Geometry: final body of the model. Coordinates: model frame, mm. A direction names the side the tool comes from. Round coordinates to 2 decimals unless told otherwise and drop trailing zeros. Order: outer loops, then holes, each group sorted by start corner. A loop starts at its lowest first (then second) coordinate and runs counter-clockwise, first axis right, second up. Notation, with made-up numbers: (71.5, -10.5) - (101.5, -10.5) arc R25 cw to (101.5, 20.5) - close; hole circle Ø11 at (12, -24). An arc over 180 degrees is marked (long way). Put each result on its own line as item: value. Start each with the question number.
(1) Section A-A (x = 0). Count the separate pieces of the cut face and the enclosed holes in it, and give its area (3 significant figures).
(2) Material intervals for L1, parallel to X at y = 2.5, z = 0; L2, parallel to Y at x = -3.5, z = 7; L3, parallel to Y at x = 0, z = 14, sorted ascending. Write a range as [from, to].
(3) Section D-D (x = 8.75). Output: boundary loops of the cut face in (y, z), and give its area (3 significant figures).
(4) Pin query (flat end, axial travel): P1, Ø8, axis at x = 2.5, z = 24.5, coming from the -Y side; P2, Ø1.5, axis at y = 3, z = 16, coming from the -X side; P3, Ø10, axis at x = -3, z = 23, coming from the +Y side. Return the tip coordinate at first contact, or that it passes through.
(5) Pull-direction query (X, two-part tool) for faces 5 (the face through (0, 1, 20)), 6 (the face through (-0.05, 5.01, -5.19)), 7 (the face through (-5.19, 5.01, 0.05)); classes: released by +X, released by -X, zero draft, split by the parting line, or undercut.
(6) Section C-C (z = -7.5). Output: boundary loops of the cut face in (x, y), and give its area (3 significant figures).
(7) Section B-B (y = 4.75). Output: boundary loops of the cut face in (x, z), and give its area (3 significant figures).
(8) Access query for faces 1 (the face through (5.272, 4.986, 5.335)), 2 (the face through (-0.1, 0.5, 9.798)), 3 (the face through (5, 2, 18)), 4 (the face through (-5.335, 4.986, 5.272)). Directions: +Z, -Z, +X, -X, +Y, -Y. A direction counts if a zero-diameter tool reaches every point of the face in a straight line with its end or side. Return the directions, or none.
from build123d import *

# Parameters (mm, degrees)
SKETCH1_R           = 11
SKETCH1_R_2         = 4.25
BOSS_EXTRUDE1_DEPTH = 4
SKETCH2_R           = 1.4
CUT_EXTRUDE1_DEPTH  = 17.062378404
SKETCH3_R           = 7.5
BOSS_EXTRUDE2_DEPTH = 2
SKETCH4_R           = 2.811136831
CUT_EXTRUDE2_DEPTH  = 2
SKETCH5_R           = 4.5
BOSS_EXTRUDE3_DEPTH = 7
CUT_EXTRUDE3_START  = -6
SKETCH6_R           = 4.5
SKETCH6_R_2         = 4
CUT_EXTRUDE3_DEPTH  = 6
BOSS_EXTRUDE4_DEPTH = 4
SKETCH11_W          = 20
SKETCH11_H          = 1
CUT_EXTRUDE5_DEPTH  = 37.234215306
FILLET1_R           = 3


with BuildPart() as part:
    # Sketch1 → Boss-Extrude1 (new body)
    with BuildSketch(Plane(origin=(0, 0, 0), x_dir=(1, 0, 0), z_dir=(0, 1, 0))):
        with Locations(Location((0, 0, 0), (0, 0, 270))):
            Circle(SKETCH1_R)
        with Locations(Location((0, 0, 0), (0, 0, 270))):
            Circle(SKETCH1_R_2, mode=Mode.SUBTRACT)
    extrude(amount=BOSS_EXTRUDE1_DEPTH)

    # Sketch2 → Cut-Extrude1 (cut, through all)
    with BuildSketch(Plane(origin=(0, 4, 0), x_dir=(1, 0, 0), z_dir=(0, 1, 0))):
        with Locations(Location((0, 8, 0), (0, 0, 270))):
            Circle(SKETCH2_R)
        with Locations(Location((8, 0, 0), (0, 0, 270))):
            Circle(SKETCH2_R)
        with Locations(Location((0, -8, 0), (0, 0, 270))):
            Circle(SKETCH2_R)
        with Locations(Location((-8, 0, 0), (0, 0, 270))):
            Circle(SKETCH2_R)
    extrude(amount=-CUT_EXTRUDE1_DEPTH, mode=Mode.SUBTRACT)

    # Sketch3 → Boss-Extrude2 (add)
    with BuildSketch(Plane(origin=(0, 4, 0), x_dir=(1, 0, 0), z_dir=(0, 1, 0))):
        with Locations(Location((0, 0, 0), (0, 0, 80.315835906))):
            Circle(SKETCH3_R)
    extrude(amount=BOSS_EXTRUDE2_DEPTH)

    # Sketch4 → Cut-Extrude2 (cut)
    with BuildSketch(Plane(origin=(0, 6, 0), x_dir=(1, 0, 0), z_dir=(0, 1, 0))):
        with Locations((8, 0)):
            Circle(SKETCH4_R)
        with Locations((0, -8)):
            Circle(SKETCH4_R)
        with Locations((-8, 0)):
            Circle(SKETCH4_R)
        with Locations((0, 8)):
            Circle(SKETCH4_R)
    extrude(amount=-CUT_EXTRUDE2_DEPTH, mode=Mode.SUBTRACT)

    # Sketch5 → Boss-Extrude3 (add)
    with BuildSketch(Plane(origin=(0, 6, 0), x_dir=(1, 0, 0), z_dir=(0, 1, 0))):
        with Locations(Location((0, 0, 0), (0, 0, 270))):
            Circle(SKETCH5_R)
    extrude(amount=BOSS_EXTRUDE3_DEPTH)

    # Sketch6 → Cut-Extrude3 (cut)
    with BuildSketch(Plane(origin=(0, 13, 0), x_dir=(1, 0, 0), z_dir=(0, 1, 0)).offset(CUT_EXTRUDE3_START)):
        with Locations(Location((0, 0, 0), (0, 0, 270))):
            Circle(SKETCH6_R)
        with Locations(Location((0, 0, 0), (0, 0, 270))):
            Circle(SKETCH6_R_2, mode=Mode.SUBTRACT)
    extrude(amount=CUT_EXTRUDE3_DEPTH, mode=Mode.SUBTRACT)

    # Sketch8 → Boss-Extrude4 (add)
    with BuildSketch(Plane.XZ):
        with BuildLine():
            Line((5, 29.797958971), (-5, 29.797958971))
            Line((-5, 29.797958971), (-5, 9.797958971))
            ThreePointArc((-5, 9.797958971), (0, 11), (5, 9.797958971))
            Line((5, 9.797958971), (5, 29.797958971))
        make_face()
    extrude(amount=-BOSS_EXTRUDE4_DEPTH)

    # Sketch11 → Cut-Extrude5 (cut, through all)
    with BuildSketch(Plane.ZY.offset(5)):
        with Locations((19.797958971, 0.5)):
            Rectangle(SKETCH11_W, SKETCH11_H)
    extrude(amount=-CUT_EXTRUDE5_DEPTH, mode=Mode.SUBTRACT)

    # Fillet1
    fillet1_edges = [part.edges().sort_by_distance(p)[0] for p in [
        (5, 2.5, 29.797958971),
        (-5, 2.5, 29.797958971),
    ]]
    fillet(fillet1_edges, radius=FILLET1_R)


solid = part.part
Checks:
1. separate pieces: 3
1. enclosed holes: 0
1. area: 165 mm²
2. L1: x = [-11, -9.4], [-6.6, -4.25], [4.25, 6.6], [9.4, 11]
2. L2: y = [0, 4]
2. L3: y = [1, 4]
3. outline: (0, -6.67) - (4, -6.67) - (4, -1.18) - (0, -1.18) - close; (0, 1.18) - (4, 1.18) - (4, 6.67) - (0, 6.67) - close
3. area: 43.9 mm²
4. P1: stops at y = 1
4. P2: stops at x = -5
4. P3: stops at y = 4
5. face 5: zero draft
5. face 6: undercut
5. face 7: released by -X
6. outline: (-8.05, 0) - (-1.31, 0) - (-1.31, 4) - (-8.05, 4) - close; (1.31, 0) - (8.05, 0) - (8.05, 4) - (1.31, 4) - close
6. area: 53.9 mm²
7. outline: (-7.02, -2.64) arc R7.5 ccw to (-2.64, -7.02) arc R2.81 cw to (2.64, -7.02) arc R7.5 ccw to (7.02, -2.64) arc R2.81 cw to (7.02, 2.64) arc R7.5 ccw to (2.64, 7.02) arc R2.81 cw to (-2.64, 7.02) arc R7.5 ccw to (-7.02, 2.64) arc R2.81 cw to start
7. area: 142 mm²
8. face 1: +Z, +X, +Y
8. face 2: +Z, +X, -X, -Y
8. face 3: +Z, +X, +Y, -Y
8. face 4: +Z, -X, +Y
